Here's the drawing with two shaded views (mm, measured from the low corner). I have some questions. Coordinates: 2 decimals unless noted, no trailing zeros. Write each loop counter-clockwise with the first axis right and the second up, starting at its lowest first coordinate (ties: lowest second). Pieces come first, ordered by that corner, then holes.
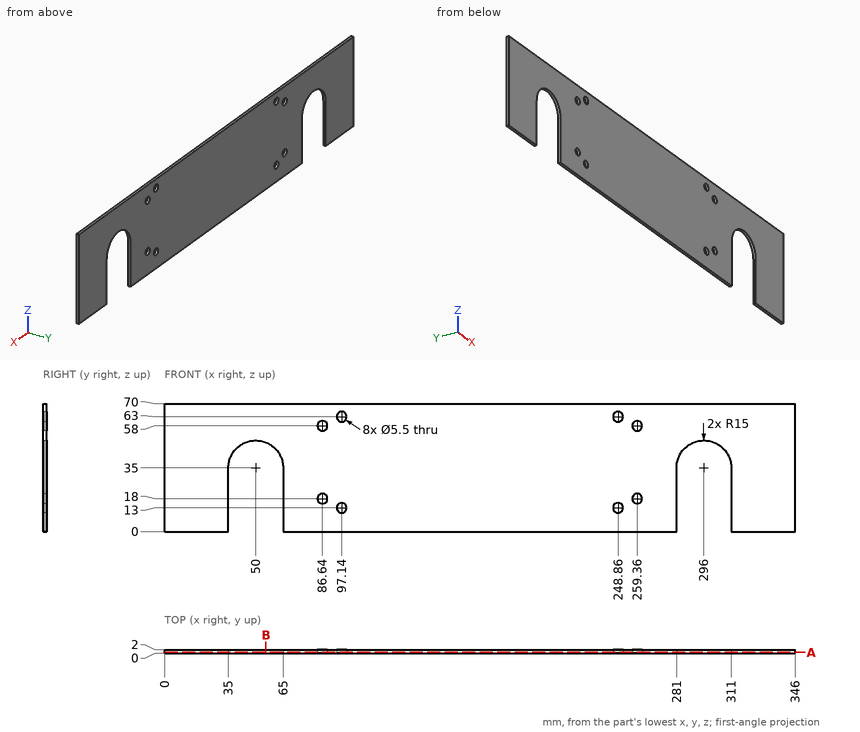
1. Please list where these lines run through material, in increasing order: line 1 along X through (y, z) = (0.5, 27); line 2 along Z through (x, y) = (259.36, 1.2); line 3 along X through (y, z) = (1.15, 61).
Verdict:
line 1: x = 0 to 35, 65 to 281, 311 to 346
line 2: z = 0 to 15.25, 20.75 to 55.25, 60.75 to 70
line 3: x = 0 to 95.25, 99.03 to 246.97, 250.75 to 346
2. I want a section at B-B on x = 55.5. Please give me the cut outline in (y, z), plus the area to 3 significant figures.
Verdict:
outline: (0, 48.96) - (2, 48.96) - (2, 70) - (0, 70) - close
area: 42.1 mm2
3. I want a section at A-A on y = 0.4. Give the number of separate pieces and of enclosed holes in the cut face, plus the area to 3 significant figures.
Verdict:
separate pieces: 1
enclosed holes: 8
area: 21,200 mm2
4. For pin 1 (4.5 mm diameter, centred on x = 86.64, z = 18, fed in from +Y), with a flat end and sliding along its axis, tell me the tip position at first contact or that it passes through.
Verdict:
pin 1: passes through
